from build123d import *

# Parameters (mm, degrees)
SKETCH1_R           = 3
BOSS_EXTRUDE1_DEPTH = 38
SKETCH2_R           = 1
CUT_EXTRUDE3_DEPTH  = 19
SKETCH4_R           = 1
CUT_EXTRUDE4_DEPTH  = 19


with BuildPart() as part:
    # Sketch1 → Boss-Extrude1 (new body)
    with BuildSketch(Plane.XY):
        Circle(SKETCH1_R)
    extrude(amount=BOSS_EXTRUDE1_DEPTH)

    # Sketch2 → Cut-Extrude3 (cut, symmetric)
    with BuildSketch(Plane(origin=(0, 0, 0), x_dir=(1, 0, 0), z_dir=(0, 1, 0))):
        with Locations(Location((0, -19, 0), (0, 0, 270))):
            Circle(SKETCH2_R)
    extrude(amount=CUT_EXTRUDE3_DEPTH, both=True, mode=Mode.SUBTRACT)

    # Sketch4 → Cut-Extrude4 (cut, symmetric)
    with BuildSketch(Plane(origin=(0, 0, 0), x_dir=(0, 0, -1), z_dir=(1, 0, 0))):
        with Locations(Location((-35, 0, 0), (0, 0, 180))):
            Circle(SKETCH4_R)
        with Locations(Location((-3, 0, 0), (0, 0, 180))):
            Circle(SKETCH4_R)
    extrude(amount=CUT_EXTRUDE4_DEPTH, both=True, mode=Mode.SUBTRACT)


solid = part.part
Can you work these out from the model? Positions are in its coordinate system, mm. Give positions to 0.01 mm unless a question says otherwise; leave off trailing zeros. Order: outer loops, then holes, each group sorted by start corner. A loop starts at its lowest first (then second) coordinate and runs counter-clockwise, first axis right, second up. Notation, with made-up numbers: M 74.5,18 L 120.5,18 A16 ccw 120.5,23 Z; hole C 72,72.5 d7. An arc over 180 degrees is marked long. Use a Markdown table: item, result. Add a question column.
Item 1: Suppose I cut it at A-A (y = 0). List the corners of the cut face in (x, z) for me, then the cut area to 3 significant figures.
Item 2: If I drill on L1, parallel to Z at x = -0.25, y = 0.5; L2, parallel to Z at x = 2, y = -0.25; L3, parallel to Y at x = -2.25, z = 35, over which ranges is the centre line in solid material (lowest first)? Write a range as [from, to].
Item 3: We'd pull the mould along X, two halves only. Please class faces 1 (the cylindrical face through (0, 0, 18)), 2 (the cylindrical face through (2.86, 0.9, 18.73)), 3 (the flat face through (0, 0, 38)): +X half, -X half, draft (parallel to the pull), parting line (faces both ways), or undercut.
Item 4: Will these pins go through, and if not, where does the flat tip stop? pin 1 (3 mm diameter, centred on y = 0, z = 35, fed in from -X); pin 2 (1.6 mm diameter, centred on x = 0, z = 19, fed in from +Y); pin 3 (2 mm diameter, centred on x = 1.5, z = 13, fed in from -Y).
Item 5: Suppose I cut it at C-C (z = 19). List the corners of the cut face in (x, y) for me.
Item 6: Suppose I cut it at D-D (y = -2.5). List the corners of the cut face in (x, z) for me, then the cut area to 3 significant figures.
Item 7: Suppose I cut it at B-B (x = -1.75). List the corners of the cut face in (y, z) for me.
Answer sheet:
| question | item | result |
|---|---|---|
| 1 | outline | M -3,0 L 3,0 L 3,2 L -3,2 Z; M -3,4 L 3,4 L 3,34 L -3,34 Z; M -3,36 L 3,36 L 3,38 L -3,38 Z; hole C 0,19 d2 |
| 1 | area | 201 mm² |
| 2 | L1 | z = [0, 2.13], [3.87, 18.03], [19.97, 34.13], [35.87, 38] |
| 2 | L2 | z = [0, 2.03], [3.97, 34.03], [35.97, 38] |
| 2 | L3 | y = [-1.98, -1], [1, 1.98] |
| 3 | face 1 | undercut |
| 3 | face 2 | parting line |
| 3 | face 3 | draft |
| 4 | pin 1 | stops at x = -3 |
| 4 | pin 2 | passes through |
| 4 | pin 3 | stops at y = -2.96 |
| 5 | outline | M -1,-2.83 L -1,2.83 A3 ccw Z; M 1,-2.83 A3 ccw 1,2.83 Z |
| 6 | outline | M -1.66,0 L 1.66,0 L 1.66,38 L -1.66,38 Z; hole C 0,19 d2 |
| 6 | area | 123 mm² |
| 7 | outline | M -2.44,0 L 2.44,0 L 2.44,38 L -2.44,38 Z; hole C 0,3 d2; hole C 0,35 d2 |
